Input: part model. Units: mm. Frame: model coordinates. Face numbers are marked on the shaded views. A direction names the side the tool comes from. Round coordinates to 2 decimals unless told otherwise and drop trailing zeros. Loops run counter-clockwise (first coordinate to the right, second up) from the corner with the lowest first, then second, coordinate; pieces in that order, holes last. Notation, with made-up numbers: (14.25, -33) - (57.25, -33) arc R14 cw to (57.25, -11) - close; hole circle Ø6 at (79.25, 6). An arc over 180 degrees is marked (long way). One line per question, with ' | ' between items. Start each with the question number.
Item 1: First-contact query: pin 1 (11 mm diameter, centred on x = -10.5, y = -19, fed in from -Z); pin 2 (17.5 mm diameter, centred on x = -11.5, y = -14, fed in from -Z); pin 3 (10 mm diameter, centred on y = 5.5, z = -23, fed in from +X); pin 4 (0.9 mm diameter, centred on x = -7.5, z = -17.5, fed in from -Y). Flat tips, straight axial feed; report the tip coordinate or a pass-through.
Item 2: Section A-A, the plane z = -2. Return loops of the section in (x, y), plus the area to 3 significant figures.
Item 3: Section C-C, the plane y = 17. Return loops of the section in (x, z), plus the area to 3 significant figures.
Item 4: Set-up query: the marked faces 1, 2, 3, 4 and 5. Return all of +Z, -Z, +X, -X, +Y, -Y with unobstructed straight access to the full face (end or side cutting, diameter ignored); none if empty.
Item 5: Material intervals for line 1 along X through (y, z) = (5, 27); line 2 along Y through (x, z) = (43, 1), sorted ascending.
Item 6: Section B-B, the plane y = -14.5. Give the number of separate pieces and of enclosed holes in the cut face, plus the area to 3 significant figures.
```python
from build123d import *

# Parameters (mm, degrees)
SKETCH1_W           = 122.936
SKETCH1_H           = 97.028
BOSS_EXTRUDE1_DEPTH = 26.162
SKETCH2_W           = 138.938
SKETCH2_H           = 97.028
BOSS_EXTRUDE2_DEPTH = 6.35
SKETCH3_W           = 3.175
SKETCH3_H           = 21.844
BOSS_EXTRUDE3_DEPTH = 138.938


with BuildPart() as part:
    # Sketch1 → Boss-Extrude1 (new body)
    with BuildSketch(Plane(origin=(0, 0, 0), x_dir=(1, 0, 0), z_dir=(0, 1, 0))):
        Rectangle(SKETCH1_W, SKETCH1_H)
    extrude(amount=BOSS_EXTRUDE1_DEPTH)

    # Sketch2 → Boss-Extrude2 (add)
    with BuildSketch(Plane.XZ):
        Rectangle(SKETCH2_W, SKETCH2_H)
    extrude(amount=BOSS_EXTRUDE2_DEPTH)

    # Sketch3 → Boss-Extrude3 (add, through all)
    with BuildSketch(Plane(origin=(69.469, 0, 0), x_dir=(0, 0, -1), z_dir=(1, 0, 0))):
        with Locations((-40.8305, -17.272)):
            Rectangle(SKETCH3_W, SKETCH3_H)
        with Locations((-46.9265, -17.272)):
            Rectangle(SKETCH3_W, SKETCH3_H)
        with Locations((-34.7345, -17.272)):
            Rectangle(SKETCH3_W, SKETCH3_H)
        with Locations((-28.6385, -17.272)):
            Rectangle(SKETCH3_W, SKETCH3_H)
        with Locations((-22.5425, -17.272)):
            Rectangle(SKETCH3_W, SKETCH3_H)
        with Locations((-16.4465, -17.272)):
            Rectangle(SKETCH3_W, SKETCH3_H)
        with Locations((-10.3505, -17.272)):
            Rectangle(SKETCH3_W, SKETCH3_H)
        with Locations((-4.2545, -17.272)):
            Rectangle(SKETCH3_W, SKETCH3_H)
        with Locations((1.8415, -17.272)):
            Rectangle(SKETCH3_W, SKETCH3_H)
        with Locations((7.9375, -17.272)):
            Rectangle(SKETCH3_W, SKETCH3_H)
        with Locations((14.0335, -17.272)):
            Rectangle(SKETCH3_W, SKETCH3_H)
        with Locations((20.1295, -17.272)):
            Rectangle(SKETCH3_W, SKETCH3_H)
        with Locations((26.2255, -17.272)):
            Rectangle(SKETCH3_W, SKETCH3_H)
        with Locations((32.3215, -17.272)):
            Rectangle(SKETCH3_W, SKETCH3_H)
        with Locations((38.4175, -17.272)):
            Rectangle(SKETCH3_W, SKETCH3_H)
        with Locations((44.5135, -17.272)):
            Rectangle(SKETCH3_W, SKETCH3_H)
    extrude(amount=-BOSS_EXTRUDE3_DEPTH)


solid = part.part
```
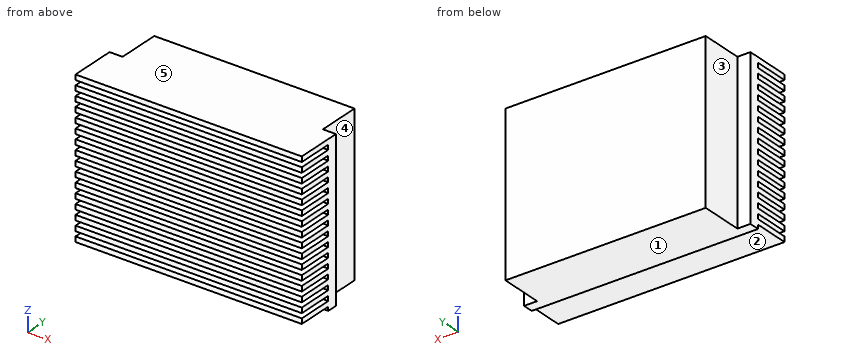
Return value:
1) pin 1: z = -46.1 | pin 2: z = -48.51 | pin 3: x = 61.47 | pin 4: y = -6.35
2) outline: (-69.47, -28.19) - (69.47, -28.19) - (69.47, 0) - (61.47, 0) - (61.47, 26.16) - (-61.47, 26.16) - (-61.47, 0) - (-69.47, 0) - close | area: 7,130 mm2
3) outline: (-61.47, -48.51) - (61.47, -48.51) - (61.47, 48.51) - (-61.47, 48.51) - close | area: 11,900 mm2
4) face 1: -Z, +X, -X, +Y, -Y | face 2: -Z, +X, -X, -Y | face 3: +Z, -Z, -X, +Y | face 4: +Z, -Z, +X, +Y | face 5: +Z, +X, -X, +Y, -Y
5) line 1: -61.47 to 61.47 | line 2: -6.35 to 26.16
6) separate pieces: 16 | enclosed holes: 0 | area: 7,060 mm2
